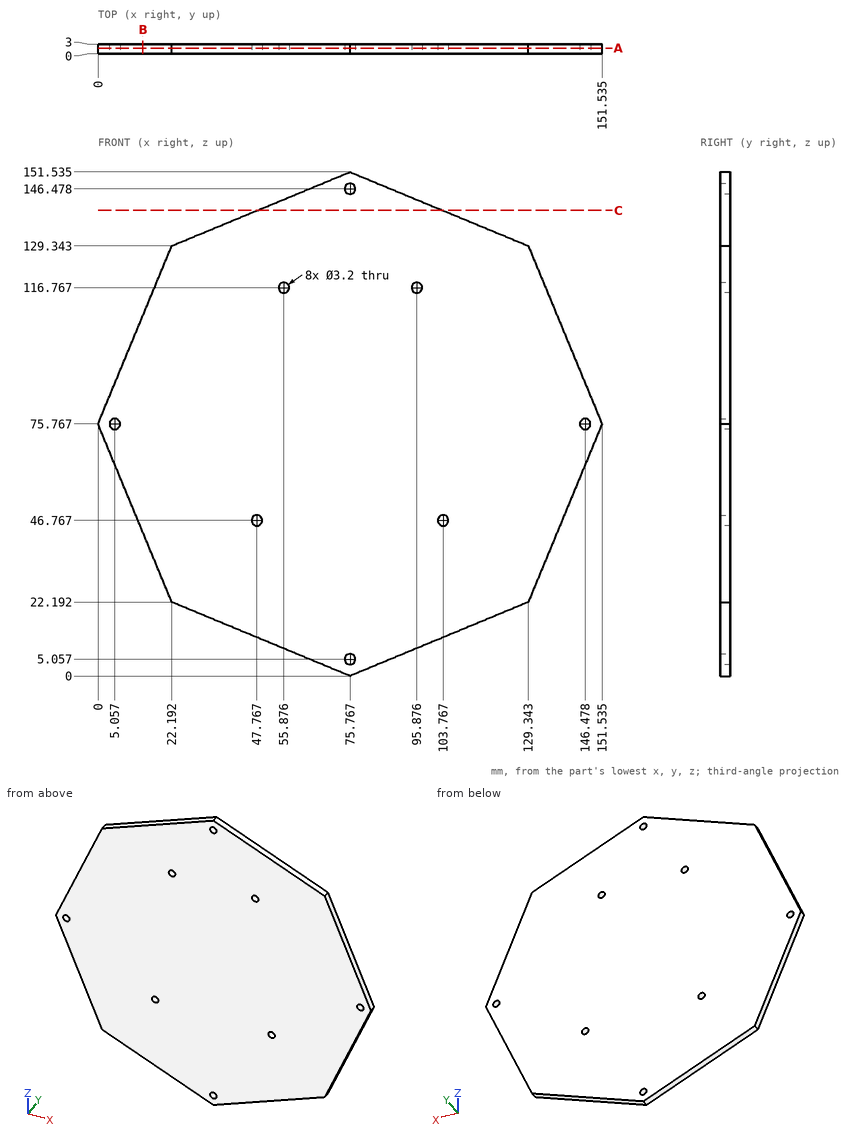
Job drawing, mm, ordinate dimensions from the low corner. One solid piece. Give positions to 0.01 mm unless a question says otherwise; leave off trailing zeros. Order: outer loops, then holes, each group sorted by start corner. A loop starts at its lowest first (then second) coordinate and runs counter-clockwise, first axis right, second up. Notation, with made-up numbers: (78, 71) - (99, 71) arc R31 cw to (99, 107) - close; hole circle Ø2 at (16.5, -16.5). An arc over 180 degrees is marked (long way). Answer in a Markdown table with one row per item.
1. Saw through at A-A, the plane y = 1.75. Count the separate pieces of the cut face and the enclosed holes in it, plus the area to 3 significant figures.
Data:
| item | result |
|---|---|
| separate pieces | 1 |
| enclosed holes | 8 |
| area | 16,200 mm² |
2. Saw through at B-B, the plane x = 13.5. Give the cut face in (y, z) (1 decimal).
Data:
| item | result |
|---|---|
| outline | (0, 43.2) - (3, 43.2) - (3, 108.4) - (0, 108.4) - close |
3. Saw through at C-C, the plane z = 140. Give the cut face in (x, y) (1 decimal).
Data:
| item | result |
|---|---|
| outline | (47.9, 0) - (103.6, 0) - (103.6, 3) - (47.9, 3) - close |
4. Flat gauge pins, fed straight in: pin 1 (3 mm diameter, centred on x = 103.77, z = 46.77, fed in from -Y); pin 2 (3.5 mm diameter, centred on x = 55.88, z = 116.77, fed in from +Y); pin 3 (1.5 mm diameter, centred on x = 108, y = 2.5, fed in from -Z); pin 4 (1 mm diameter, centred on y = 1, z = 73, fed in from +X) (1 decimal). Where does each tip first touch, or does it go through?
Data:
| item | result |
|---|---|
| pin 1 | passes through |
| pin 2 | stops at y = 3 |
| pin 3 | stops at z = 13.04 |
| pin 4 | stops at x = 150.6 |
5. Probe probe 1 along Z at (x, y) = (66, 2.25) (1 decimal); probe 2 along X at (y, z) = (0.4, 66.5) (1 decimal); probe 3 along X at (y, z) = (1.35, 87.5) (1 decimal). List the from-to ranges inside material, lowest first. Write a range as [from, to].
Data:
| item | result |
|---|---|
| probe 1 | z = [4, 147.5] |
| probe 2 | x = [3.8, 147.7] |
| probe 3 | x = [4.9, 146.7] |
